Check sheet for the drawn part. Datum: minimum x, y, z corner. Units: mm. A direction names the side the tool comes from. Round coordinates to 2 decimals unless told otherwise and drop trailing zeros. Write each loop counter-clockwise with the first axis right and the second up, starting at its lowest first coordinate (ties: lowest second). Pieces come first, ordered by that corner, then holes.
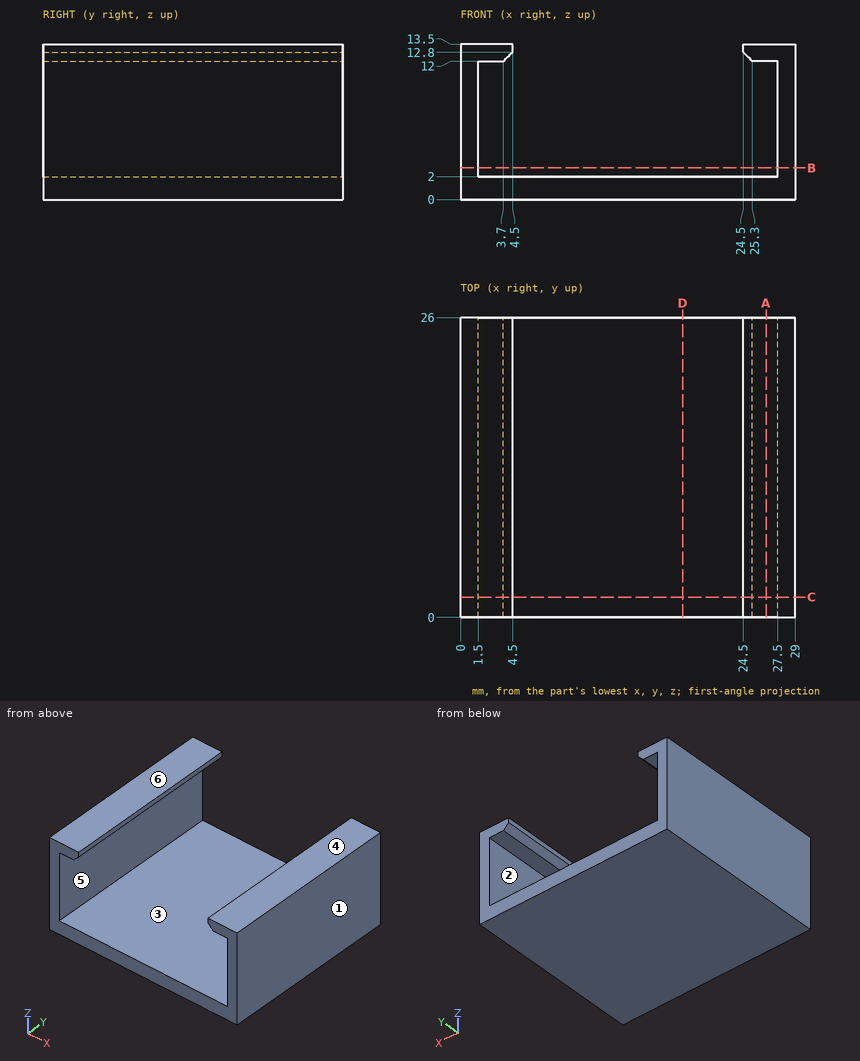
1. Set-up check for the marked faces 5 and 6: record each of +Z, -Z, +X, -X, +Y, -Y from which the full face is reachable in a straight line by a thin tool's end or side.
2. Go/stop test with flat-tipped pins: pin 1 (4 mm diameter, centred on x = 14.5, y = 13.5, fed in from +Z); pin 2 (5 mm diameter, centred on x = 24.5, z = 7, fed in from +Y). Record where each tip stops, or that it passes through.
3. Sectioned sample at C-C, the plane y = 1.75. Enter the section's corners in (x, z).
4. Sectioned sample at A-A, the plane x = 26.5. Enter the section's corners in (y, z).
5. Scan lines: line 1 along X through (y, z) = (18.25, 3.5); line 2 along Z through (x, y) = (26.5, 21.5); line 3 along Z through (x, y) = (16.25, 19.5). Record each from-to range of solid material in increasing order.
6. Sectioned sample at D-D, the plane x = 19.25. Enter the section's corners in (y, z).
7. Release check for a two-part mould opening along X. For the marked faces 1, 2, 3 and 4 record: released by +X, released by -X, zero draft, split by the parting line, or undercut.
8. Sectioned sample at B-B, the plane z = 2.75. Enter the section's corners in (x, y), plus the area to 3 significant figures.
Computed values:
1. face 5: +Y, -Y
1. face 6: +Z, +X, -X, +Y, -Y
2. pin 1: stops at z = 2
2. pin 2: passes through
3. outline: (0, 0) - (29, 0) - (29, 13.5) - (24.5, 13.5) - (24.5, 12.8) - (25.3, 12) - (27.5, 12) - (27.5, 2) - (1.5, 2) - (1.5, 12) - (3.7, 12) - (4.5, 12.8) - (4.5, 13.5) - (0, 13.5) - close
4. outline: (0, 0) - (26, 0) - (26, 2) - (0, 2) - close; (0, 12) - (26, 12) - (26, 13.5) - (0, 13.5) - close
5. line 1: x = 0 to 1.5, 27.5 to 29
5. line 2: z = 0 to 2, 12 to 13.5
5. line 3: z = 0 to 2
6. outline: (0, 0) - (26, 0) - (26, 2) - (0, 2) - close
7. face 1: released by +X
7. face 2: undercut
7. face 3: undercut
7. face 4: zero draft
8. outline: (0, 0) - (1.5, 0) - (1.5, 26) - (0, 26) - close; (27.5, 0) - (29, 0) - (29, 26) - (27.5, 26) - close
8. area: 78.0 mm2
